Part print with two shaded views. Sizes in mm from the minimum x, y, z corner. A direction names the side the tool comes from. Round coordinates to 2 decimals unless told otherwise and drop trailing zeros. Loops run counter-clockwise (first coordinate to the right, second up) from the corner with the lowest first, then second, coordinate; pieces in that order, holes last. Notation, with made-up numbers: (1, -37) - (22, -37) arc R17 ccw to (22, -32) - close; hole circle Ø11 at (39, -35.75). An arc over 180 degrees is marked (long way). One line per question, with ' | ' between items.
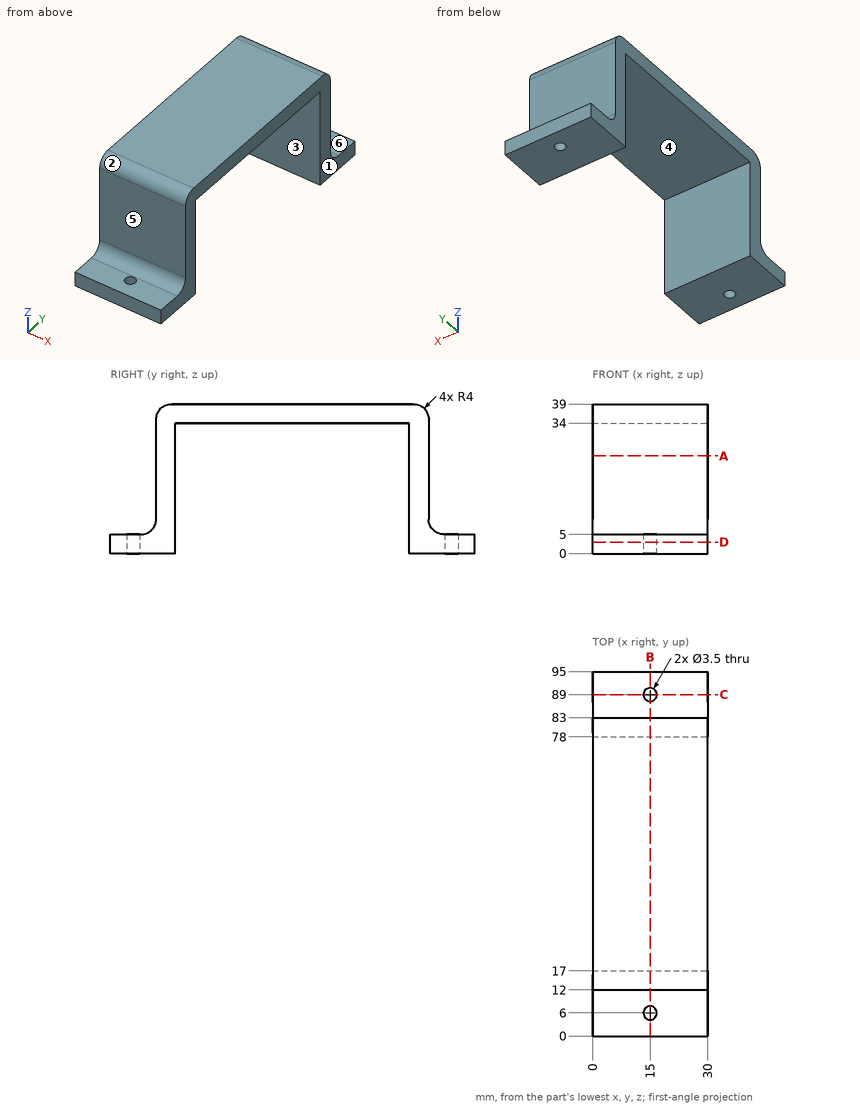
(1) Tool access for the marked faces 4, 5 and 6: list every direction of +Z, -Z, +X, -X, +Y, -Y with a clear straight run to the whole face (end or side of a thin tool).
Results found:
face 4: -Z, +X, -X | face 5: +Z, +X, -X, -Y | face 6: +Z, +X, -X, +Y
(2) Cut at C-C, the plane y = 89. Write the cut outline in (x, z), then the cut area to 4 significant figures.
Results found:
outline: (0, 0) - (13.25, 0) - (13.25, 5) - (0, 5) - close; (16.75, 0) - (30, 0) - (30, 5) - (16.75, 5) - close | area: 132.5 mm²
(3) Cut at D-D, the plane z = 3. Write the cut outline in (x, y), then the cut area to 3 significant figures.
Results found:
outline: (0, 0) - (30, 0) - (30, 17) - (0, 17) - close; (0, 78) - (30, 78) - (30, 95) - (0, 95) - close; hole circle Ø3.5 at (15, 6); hole circle Ø3.5 at (15, 89) | area: 1,000 mm²
(4) Cut at A-A, the plane z = 25.5. Write the cut outline in (x, y), then the cut area to 3 significant figures.
Results found:
outline: (0, 12) - (30, 12) - (30, 17) - (0, 17) - close; (0, 78) - (30, 78) - (30, 83) - (0, 83) - close | area: 300 mm²
(5) Probe L1, parallel to Y at x = 15, z = 3; L2, parallel to X at y = 89, z = 2.15; L3, parallel to Y at x = 18.25, z = 15. List the from-to ranges inside material, lowest first.
Results found:
L1: y = 0 to 4.25, 7.75 to 17, 78 to 87.25, 90.75 to 95 | L2: x = 0 to 13.25, 16.75 to 30 | L3: y = 12 to 17, 78 to 83
(6) Cut at B-B, the plane x = 15. Write the cut outline in (y, z), then the cut area to 3 significant figures.
Results found:
outline: (0, 0) - (4.25, 0) - (4.25, 5) - (0, 5) - close; (7.75, 0) - (17, 0) - (17, 34) - (78, 34) - (78, 0) - (87.25, 0) - (87.25, 5) - (87, 5) arc R4 cw to (83, 9) - (83, 35) arc R4 ccw to (79, 39) - (16, 39) arc R4 ccw to (12, 35) - (12, 9) arc R4 cw to (8, 5) - (7.75, 5) - close; (90.75, 0) - (95, 0) - (95, 5) - (90.75, 5) - close | area: 780 mm²
(7) Two-plate mould, pull along Y, no slides. Class the marked faces 1, 2 and 3: released by +Y, released by -Y, zero draft, split by the parting line, or undercut.
Results found:
face 1: zero draft | face 2: released by -Y | face 3: undercut
(8) Drop flat-ended pins along their axis: P1, Ø2.5, axis at x = 16, y = 92.5, coming from the +Z side; P2, Ø10, axis at x = 11.5, z = 31, coming from the +Y side; P3, Ø8, axis at x = 15, z = 11.5, coming from the +Y side. Give the stop position or say it passes through.
Results found:
P1: stops at z = 5 | P2: stops at y = 83 | P3: stops at y = 83.29
